Geometry check sheet. Reference: the model listing, model coordinates, mm. A direction names the side the tool comes from. Round coordinates to 2 decimals unless told otherwise and drop trailing zeros. Write each loop counter-clockwise with the first axis right and the second up, starting at its lowest first coordinate (ties: lowest second). Pieces come first, ordered by that corner, then holes. Notation, with made-up numbers: M -10.75,75 L 16.25,75 A23 ccw 16.25,101 Z; hole C 15.5,47.5 d9. An arc over 180 degrees is marked long. Use a Markdown table: item, result.
```python
from build123d import *

# Parameters (mm, degrees)
BOSS_EXTRU_2_DEPTH              = 1
EXTRU_MINCE1_DEPTH              = 1.5
EXTRU_MINCE1_DRAFT              = -10
ENL_V_DE_MAT_EXTRU_MINCE1_DEPTH = 101.734373448
ESQUISSE7_W                     = 5.2
ESQUISSE7_H                     = 4.1
BOSS_EXTRU_5_DEPTH              = 1.5
ESQUISSE8_W                     = 10
ESQUISSE8_H                     = 2
BOSS_EXTRU_6_DEPTH              = 2.2
CHANFREIN1_SIZE                 = 2.2
ESQUISSE9_W                     = 1.2
ESQUISSE9_H                     = 2
BOSS_EXTRU_7_DEPTH              = 2


with BuildPart() as part:
    # Esquisse2 → Boss.-Extru.2 (new body)
    with BuildSketch(Plane(origin=(0, 0, 0), x_dir=(1, 0, 0), z_dir=(0, 1, 0))):
        Polygon((-68.262395693, 28.744645862), (-59.024791386, 44.744645862), (59.024791386, 44.744645862), (68.262395693, 28.744645862), (9.237604307, -73.489291724), (-9.237604307, -73.489291724), align=None)
    extrude(amount=BOSS_EXTRU_2_DEPTH)


with BuildPart() as extru_mince1_tool:
    # Esquisse5 → Extru.-Mince1 (with draft: the straight prism first)
    with BuildSketch(Plane(origin=(0, 1, 0), x_dir=(1, 0, 0), z_dir=(0, 1, 0))):
        Polygon((-68.262395693, 28.744645862), (-9.237604307, -73.489291724), (9.237604307, -73.489291724), (68.262395693, 28.744645862), (59.024791386, 44.744645862), (-59.024791386, 44.744645862), align=None)
        Polygon((-66.299404778, 28.744645862), (-8.256108849, -71.789291724), (8.256108849, -71.789291724), (66.299404778, 28.744645862), (58.043295928, 43.044645862), (-58.043295928, 43.044645862), align=None, mode=Mode.SUBTRACT)
    extrude(amount=EXTRU_MINCE1_DEPTH)
    # Extru.-Mince1: the draft: its side faces are tilted about the plane it starts from
    extru_mince1_sides = [extru_mince1_tool.faces().sort_by_distance(p)[0] for p in [
        (-38.75, 1.75, 22.372322931),
        (0, 1.75, 73.489291724),
        (38.75, 1.75, 22.372322931),
        (63.643593539, 1.75, -36.744645862),
        (0, 1.75, -44.744645862),
        (-63.643593539, 1.75, -36.744645862),
        (-62.171350353, 1.75, -35.894645862),
        (0, 1.75, -43.044645862),
        (62.171350353, 1.75, -35.894645862),
        (37.277756814, 1.75, 21.522322931),
        (0, 1.75, 71.789291724),
        (-37.277756814, 1.75, 21.522322931),
    ]]
    draft(extru_mince1_sides, Plane(origin=(0, 1, 0), x_dir=(1, 0, 0), z_dir=(0, 1, 0)), EXTRU_MINCE1_DRAFT)


with BuildPart() as part_1:
    add(part.part)

    # Extru.-Mince1: add extru_mince1_tool
    add(extru_mince1_tool.part)

    # Esquisse6 → Enlèv. de mat.-Extru.-Mince1 (cut, through all)
    with BuildSketch(Plane.XZ):
        Polygon((-59.89081679, -46.244645862), (59.89081679, -46.244645862), (69.994446501, -28.744645862), (10.103629711, 74.989291724), (-10.103629711, 74.989291724), (-69.994446501, -28.744645862), align=None)
        Polygon((-59.024791386, -44.744645862), (59.024791386, -44.744645862), (68.262395693, -28.744645862), (9.237604307, 73.489291724), (-9.237604307, 73.489291724), (-68.262395693, -28.744645862), align=None, mode=Mode.SUBTRACT)
    extrude(amount=-ENL_V_DE_MAT_EXTRU_MINCE1_DEPTH, mode=Mode.SUBTRACT)

    # Esquisse7 → Boss.-Extru.5 (add)
    with BuildSketch(Plane(origin=(0, 1, 0), x_dir=(1, 0, 0), z_dir=(0, 1, 0))):
        with Locations((0, 42.694645862)):
            Rectangle(ESQUISSE7_W, ESQUISSE7_H)
        Polygon((33.899295844, -22.573988981), (36.499295844, -18.070656881), (40.05, -20.120656881), (37.45, -24.623988981), align=None)
        Polygon((-36.499295844, -18.070656881), (-33.899295844, -22.573988981), (-37.45, -24.623988981), (-40.05, -20.120656881), align=None)
    extrude(amount=BOSS_EXTRU_5_DEPTH)

    # Esquisse8 → Boss.-Extru.6 (add)
    with BuildSketch(Plane(origin=(0, 1, 0), x_dir=(1, 0, 0), z_dir=(0, 1, 0))):
        with Locations((0, 39.644645862)):
            Rectangle(ESQUISSE8_W, ESQUISSE8_H)
        Polygon((37.699295844, -15.992195912), (32.699295844, -24.65244995), (30.967245037, -23.65244995), (35.967245037, -14.992195912), align=None)
        Polygon((-32.699295844, -24.65244995), (-37.699295844, -15.992195912), (-35.967245037, -14.992195912), (-30.967245037, -23.65244995), align=None)
    extrude(amount=BOSS_EXTRU_6_DEPTH)

    # Chanfrein1
    chanfrein1_edges = [part_1.edges().sort_by_distance(p)[0] for p in [
        (-31.833270441, 1, 24.15244995),
        (-36.833270441, 1, 15.492195912),
        (-33.467245037, 1, 19.322322931),
        (36.833270441, 1, 15.492195912),
        (33.467245037, 1, 19.322322931),
        (31.833270441, 1, 24.15244995),
        (5, 1, -39.644645862),
        (-5, 1, -39.644645862),
        (0, 1, -38.644645862),
    ]]
    chamfer(chanfrein1_edges, length=CHANFREIN1_SIZE - 0.0001)  # a hair under: the kernel refuses the full size

    # Esquisse9 → Boss.-Extru.7 (add)
    with BuildSketch(Plane(origin=(0, 3.2, 0), x_dir=(1, 0, 0), z_dir=(0, 1, 0))):
        with Locations((0, 39.644645862)):
            Rectangle(ESQUISSE9_W, ESQUISSE9_H)
        Polygon((34.899295844, -20.841938173), (35.499295844, -19.802707689), (33.767245037, -18.802707689), (33.167245037, -19.841938173), align=None)
        Polygon((-35.499295844, -19.802707689), (-34.899295844, -20.841938173), (-33.167245037, -19.841938173), (-33.767245037, -18.802707689), align=None)
    extrude(amount=BOSS_EXTRU_7_DEPTH)


solid = part_1.part
```
Item 1: Access from +Z, -Z, +X, -X, +Y, -Y to the whole of each face (thin tool, end or side, straight path). Record for faces 1 (the face through (-33, 3.2, 22)), 2 (the face through (52.132, 1.74, -4.466)), 3 (the face through (0, 3, -40.645)).
Outcome:
| item | result |
|---|---|
| face 1 | +Z, +Y |
| face 2 | none |
| face 3 | +Y |
Item 2: Mould release check, pull along X, two halves, no side actions. Record for faces 4 (the face through (63.579, 1.232, -36.857)), 5 (the face through (36, 3.2, 17)), 6 (the face through (32.48, 2.12, 18.87)): +X half, -X half, draft (parallel to the pull), parting line (faces both ways), or undercut.
Outcome:
| item | result |
|---|---|
| face 4 | +X half |
| face 5 | draft |
| face 6 | undercut |
Item 3: Go/stop test with flat-tipped pins: pin 1 (1.2 mm diameter, centred on y = 2, z = -41.5, fed in from +X); pin 2 (1.6 mm diameter, centred on y = 4.5, z = -39.5, fed in from -X); pin 3 (3 mm diameter, centred on x = 32.5, z = 23, fed in from +Y). Record where each tip stops, or that it passes through.
Outcome:
| item | result |
|---|---|
| pin 1 | stops at x = 61.24 |
| pin 2 | stops at x = -0.6 |
| pin 3 | stops at y = 3.2 |
Item 4: Cross-section at B-B, the plane z = 8. Record the cut outline in (x, y).
Outcome:
| item | result |
|---|---|
| outline | M -47.05,0 L 47.05,0 L 47.05,2.5 L 44.78,2.5 L 45.08,1 L -45.08,1 L -44.78,2.5 L -47.05,2.5 Z |
Item 5: Cross-section at A-A, the plane x = 44.5. Record the cut outline in (y, z), and give its area (3 significant figures).
Outcome:
| item | result |
|---|---|
| outline | M 0,-44.74 L 2.5,-44.74 L 2.5,-42.78 L 1,-43.04 L 1,9.01 L 2.5,8.48 L 2.5,12.41 L 0,12.41 Z |
| area | 65.4 mm2 |
Item 6: Material ranges on line 1 along Y through (x, z) = (39, 11); line 2 along Z through (x, y) = (-14, 1.35); line 3 along Z through (x, y) = (22, 1.8), recorded low to high. Write a range as from..to.
Outcome:
| item | result |
|---|---|
| line 1 | y = 0..1 |
| line 2 | z = -44.74..-42.98, 61.72..65.24 |
| line 3 | z = -44.74..-42.9, 47.7..51.38 |
